Design review of the part shown in the three views and the two pictorial views. Dimensions are in mm from the part's minimum x, y and z. A direction names the side the tool comes from. Give positions to 0.01 mm unless a question says otherwise; leave off trailing zeros. Loops run counter-clockwise (first coordinate to the right, second up) from the corner with the lowest first, then second, coordinate; pieces in that order, holes last.
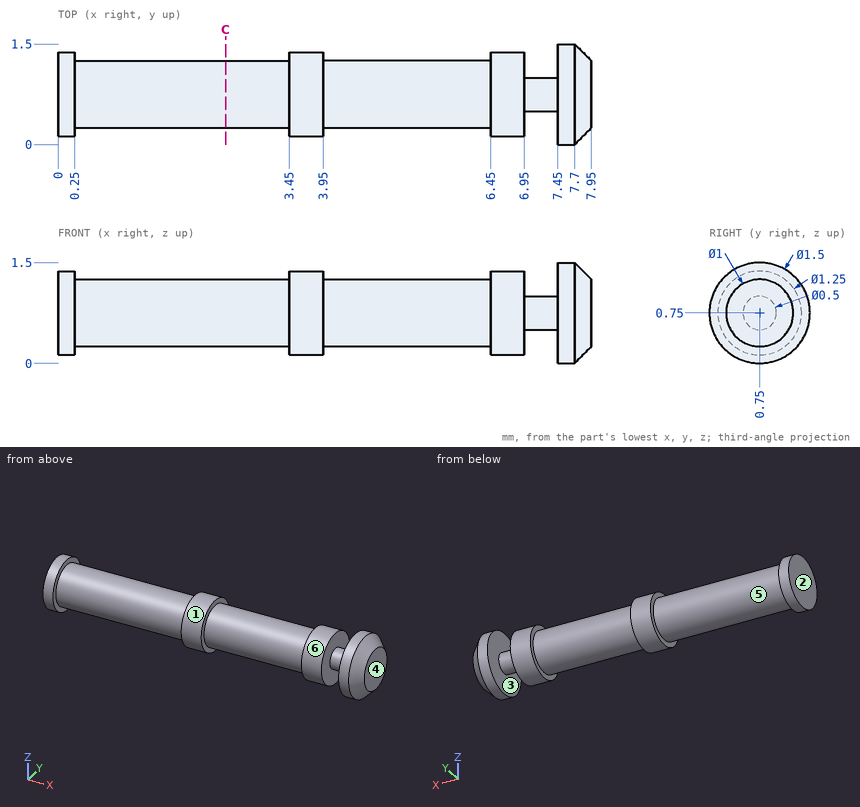
Q1. Tool access review of the marked faces 1, 2 and 3: name each direction out of +Z, -Z, +X, -X, +Y, -Y from which nothing blocks a thin tool from reaching the whole face with its end or side.
Results:
face 1: -X
face 2: +Z, -Z, -X, +Y, -Y
face 3: none
Q2. Take a section at C-C (x = 2.5). Give the boundary of the cut face in (y, z).
Results:
outline: circle Ø1 at (0.75, 0.75)
Q3. Draft analysis for pull direction X (two halves, no side actions). For the marked faces 4, 5 and 6, state which applies: pulls with the +X half, pulls with the -X half, needs draft (parallel to the pull), parting line crosses it, or undercut.
Results:
face 4: pulls with the +X half
face 5: undercut
face 6: needs draft
Q4. Wall thickness on line 1 (X direction, y = 0.75, z = 1.2); line 2 (X direction, y = 0.2, z = 0.9); line 3 (Z direction, x = 4.75, y = 0.8): over which ranges is each line inside the solid? List them lowest first.
Results:
line 1: x = 0 to 6.95, 7.45 to 7.95
line 2: x = 0 to 0.25, 3.45 to 3.95, 6.45 to 6.95, 7.45 to 7.88
line 3: z = 0.25 to 1.25
